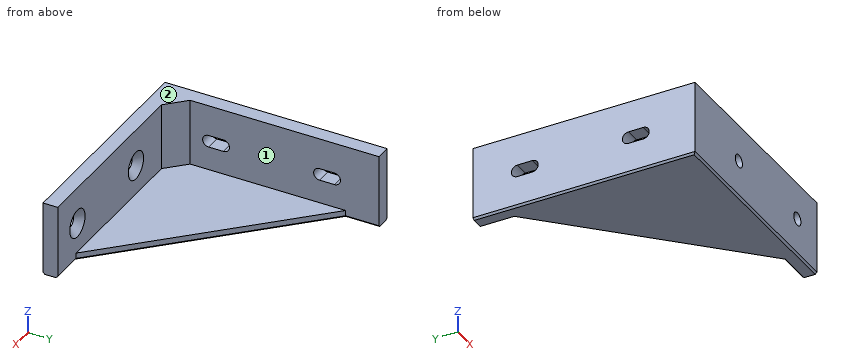
```python
from build123d import *

# Parameters (mm, degrees)
PAD_DEPTH       = 20
PAD001_DEPTH    = 2
CHAMFER_SIZE    = 0.5
CHAMFER001_SIZE = 0.5
CHAMFER002_SIZE = 0.5
CHAMFER003_SIZE = 5
SKETCH002_R     = 1.75
HOLE_DEPTH      = 25
CHAMFER004_SIZE = 2
POCKET_DEPTH    = 5
CHAMFER005_SIZE = 0.5


with BuildPart() as part:
    # Sketch → Pad (new body)
    with BuildSketch(Plane.XY):
        Polygon((0, 0), (0, 60), (4, 60), (4, 4), (60, 4), (60, 0), align=None)
    extrude(amount=PAD_DEPTH)

    # Sketch001 (on Face7 of Pad) → Pad001 (join)
    with BuildSketch(Plane(origin=(0, 0, 0), x_dir=(1, 0, 0), z_dir=(0, 0, -1))):
        Polygon((0, 0), (0, -55), (55, 0), align=None)
    extrude(amount=-PAD001_DEPTH)

    # Chamfer
    chamfer_edges = [part.edges().sort_by_distance(p)[0] for p in [
        (27.5, 0, 0),
        (57.5, 0, 0),
    ]]
    chamfer(chamfer_edges, length=CHAMFER_SIZE)

    # Chamfer001
    chamfer001_edges = [part.edges().sort_by_distance(p)[0] for p in [
        (0, 27.75, 0),
        (0, 57.5, 0),
    ]]
    chamfer(chamfer001_edges, length=CHAMFER001_SIZE)

    # Chamfer002
    chamfer002_edges = [part.edges().sort_by_distance(p)[0] for p in [
        (4, 55.5, 0),
        (55.5, 4, 0),
    ]]
    chamfer(chamfer002_edges, length=CHAMFER002_SIZE)

    # Chamfer003
    chamfer003_edges = [part.edges().sort_by_distance(p)[0] for p in [
        (4, 4, 11),
    ]]
    chamfer(chamfer003_edges, length=CHAMFER003_SIZE)

    # Sketch002 (on Face9 of Chamfer003) → Hole (cut)
    with BuildSketch(Plane(origin=(0, 4, 0), x_dir=(-1, 0, 0), z_dir=(0, 1, 0))):
        with Locations((-50.342533, 10)):
            Circle(SKETCH002_R)
        with Locations((-21.578398, 10)):
            Circle(SKETCH002_R)
    extrude(amount=-HOLE_DEPTH, mode=Mode.SUBTRACT)

    # Chamfer004
    chamfer004_edges = [part.edges().sort_by_distance(p)[0] for p in [
        (19.828398, 4, 10),
        (48.592533, 4, 10),
    ]]
    chamfer(chamfer004_edges, length=CHAMFER004_SIZE)

    # Sketch003 (on Face14 of Chamfer004) → Pocket (cut)
    with BuildSketch(Plane(origin=(0, 0, 0), x_dir=(0, -1, 0), z_dir=(-1, 0, 0))):
        with BuildLine():
            ThreePointArc((-48, 11.625), (-49.625, 10), (-48, 8.375))
            Line((-48, 8.375), (-44, 8.375))
            ThreePointArc((-44, 8.375), (-42.375, 10), (-44, 11.625))
            Line((-48, 11.625), (-44, 11.625))
        make_face()
        with BuildLine():
            ThreePointArc((-18, 11.625), (-19.625, 10), (-18, 8.375))
            Line((-18, 8.375), (-14, 8.375))
            ThreePointArc((-14, 8.375), (-12.375, 10), (-14, 11.625))
            Line((-18, 11.625), (-14, 11.625))
        make_face()
    extrude(amount=-POCKET_DEPTH, mode=Mode.SUBTRACT)

    # Chamfer005
    chamfer005_edges = [part.edges().sort_by_distance(p)[0] for p in [
        (27.5, 27.5, 0),
    ]]
    chamfer(chamfer005_edges, length=CHAMFER005_SIZE)


solid = part.part
```
Can you work these out from the model? Positions are in its coordinate system, mm. Face numbers are marked on the shaded views. A direction names the side the tool comes from. Give positions to 0.01 mm unless a question says otherwise; leave off trailing zeros. Order: outer loops, then holes, each group sorted by start corner. A loop starts at its lowest first (then second) coordinate and runs counter-clockwise, first axis right, second up. Notation, with made-up numbers: (20, 16.5) - (72, 16.5) arc R10 ccw to (72, 23.5) - close; hole circle Ø11 at (3.5, 75.25). An arc over 180 degrees is marked (long way). Use a Markdown table: item, result. Add a question column.
Q1. On a 3-axis mill with a long thin cutter (end or side, diameter ignored), from which of +Z, -Z, +X, -X, +Y, -Y can I reach the whole of each face in a straight line? I mean the marked faces 1 and 2. Say none if no direction works.
Q2. I'm going to push flat-ended pins straight in: pin 1 (23.5 mm diameter, centred on x = 26, y = 31, fed in from +Z); pin 2 (4 mm diameter, centred on x = 21.58, z = 10, fed in from -Y); pin 3 (4 mm diameter, centred on x = 50.34, z = 10, fed in from +Y); pin 4 (6 mm diameter, centred on x = 38, z = 15.5, fed in from +Y). Where does each tip first touch, or does it pass through?
Q3. If we section it at B-B on x = 31: Write out the boundary of the cut face in (y, z).
Q4. If we section it at C-C on z = 17: Write out the boundary of the cut face in (x, y).
Q5. Please list where these lines run through material, in increasing order: line 1 along X through (y, z) = (50.5, 13.5); line 2 along Z through (x, y) = (5, 41.5).
Q6. If we section it at A-A on z = 10: Write out the boundary of the cut face in (x, y) (3 decimals).
Answers follow:
| question | item | result |
|---|---|---|
| 1 | face 1 | +Z, +X, +Y |
| 1 | face 2 | +Z, +X, -X, +Y, -Y |
| 2 | pin 1 | stops at z = 2 |
| 2 | pin 2 | stops at y = 0 |
| 2 | pin 3 | stops at y = 2.25 |
| 2 | pin 4 | stops at y = 4 |
| 3 | outline | (0, 0.5) - (0.5, 0) - (23.29, 0) - (24, 0.5) - (24, 2) - (4, 2) - (4, 20) - (0, 20) - close |
| 4 | outline | (0, 0) - (60, 0) - (60, 4) - (9, 4) - (4, 9) - (4, 60) - (0, 60) - close |
| 5 | line 1 | x = 0 to 4 |
| 5 | line 2 | z = 0 to 2 |
| 6 | outline | (0, 0) - (19.828, 0) - (19.828, 2) - (17.828, 4) - (9, 4) - (4, 9) - (4, 12.375) - (0, 12.375) - close; (0, 19.625) - (4, 19.625) - (4, 42.375) - (0, 42.375) - close; (0, 49.625) - (4, 49.625) - (4, 60) - (0, 60) - close; (23.328, 0) - (48.593, 0) - (48.593, 2) - (46.593, 4) - (25.328, 4) - (23.328, 2) - close; (52.093, 0) - (60, 0) - (60, 4) - (54.093, 4) - (52.093, 2) - close |
